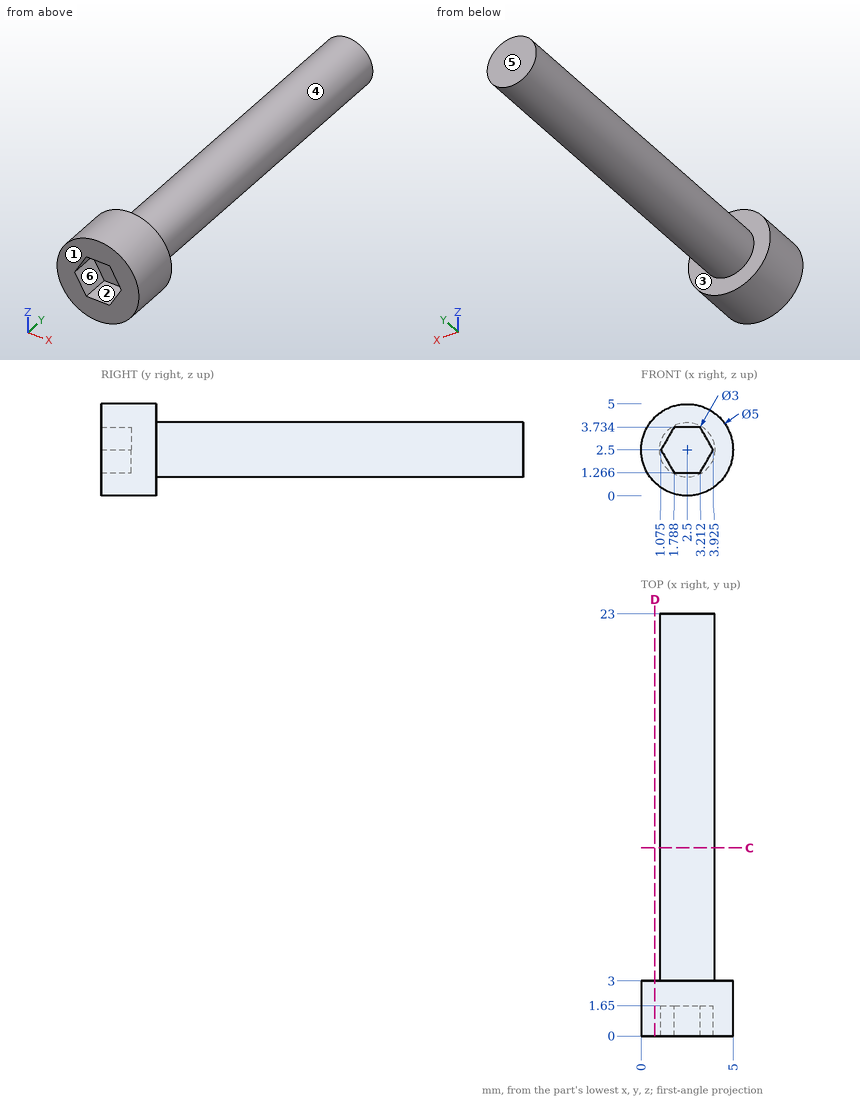
Geometry: see drawing. Coordinates: mm, zero at the bounding-box minimum. A direction names the side the tool comes from. Round coordinates to 2 decimals unless told otherwise and drop trailing zeros. Order: outer loops, then holes, each group sorted by start corner. A loop starts at its lowest first (then second) coordinate and runs counter-clockwise, first axis right, second up. Notation, with made-up numbers: (-20, 58.25) -> (25, 58.25) arc R23 ccw to (25, 77.25) -> close; hole circle Ø4 at (-13.5, 0). An arc over 180 degrees is marked (long way). Use CSV: the item, a comma, the result in double quotes.
(1) Access query for the marked faces 1, 2 and 3. Directions: +Z, -Z, +X, -X, +Y, -Y. A direction counts if a zero-diameter tool reaches every point of the face in a straight line with its end or side. Return the directions, or none.
Report:
face 1,"+Z, -Z, +X, -X, -Y"
face 2,"-Y"
face 3,"+Y"
(2) Ray query, L1, parallel to Z at x = 1.65, y = 18.75 (1 decimal); L2, parallel to Y at x = 1, z = 1.25; L3, parallel to Y at x = 2.4, z = 3.3. Return the intervals inside material, ascending.
Report:
L1,"1.3 to 3.7"
L2,"0 to 3"
L3,"1.65 to 23"
(3) First-contact query: pin 1 Ø2 at (y, z) = (17.5, 2.5) entering from +X; pin 2 Ø1.5 at (x, y) = (2, 8.5) entering from -Z. Flat tips, straight axial feed; report the tip coordinate or a pass-through.
Report:
pin 1,"x = 4"
pin 2,"z = 1"
(4) Section D-D on x = 0.75. Return the cut outline in (y, z) (1 decimal), and give its area (3 significant figures).
Report:
outline,"(0, 0.7) -> (3, 0.7) -> (3, 4.3) -> (0, 4.3) -> close"
area,"10.7 mm^2"
(5) Section C-C on y = 10.25. Return the cut outline in (x, z).
Report:
outline,"circle Ø3 at (2.5, 2.5)"
(6) Pull-direction query (X, two-part tool) for the marked faces 4, 5 and 6; classes: +X half, -X half, draft (parallel to the pull), parting line (faces both ways), or undercut.
Report:
face 4,"parting line"
face 5,"draft"
face 6,"undercut"
